```python
from build123d import *

# Parameters (mm, degrees)
F1_DEPTH  = 76.2
F1_FACE_W = 152.4
F1_FACE_H = 152.4
F2_DEPTH  = 25.4
F3_R      = 12.123607
F4_DEPTH  = 76.201
F6_DEPTH  = 28.794128
F8_DEPTH  = 25.401


with BuildPart() as f1:
    # F0 (on Front) → F1 (new body, symmetric)
    with BuildSketch(Plane.XZ):
        Polygon((-76.2, 0), (0, 0), (0, 152.4), (-25.4, 152.4), (-25.4, 28.793128), (-76.2, 28.793128), align=None)
    extrude(amount=F1_DEPTH, both=True)

    # F1_face (on face) → F2 (cut)
    with BuildSketch(Plane(origin=(0, 0, 76.2), x_dir=(0, 1, 0), z_dir=(1, 0, 0))):
        Rectangle(F1_FACE_W, F1_FACE_H)
    extrude(amount=F2_DEPTH, mode=Mode.SUBTRACT)

    # F3 (on face) → F4 (cut, through all)
    with BuildSketch(Plane.YZ):
        with Locations((0, 123.985767)):
            Circle(F3_R)
    extrude(amount=-F4_DEPTH, mode=Mode.SUBTRACT)

    # F5 (on face) → F6 (cut, through all)
    with BuildSketch(Plane.XY.offset(28.793128)):
        with BuildLine():
            Line((-63.5, 12.7), (-76.2, 12.7))
            Line((-76.2, 12.7), (-76.2, -12.7))
            Line((-76.2, -12.7), (-63.5, -12.7))
            ThreePointArc((-63.5, -12.7), (-50.8, 0), (-63.5, 12.7))
        make_face()
    extrude(amount=-F6_DEPTH, mode=Mode.SUBTRACT)

    # F7 (on face) → F8 (cut, through all)
    with BuildSketch(Plane(origin=(-25.4, 0, 0), x_dir=(0, -1, 0), z_dir=(-1, 0, 0))):
        with BuildLine():
            ThreePointArc((38.1, 152.4), (65.040768, 141.240768), (76.2, 114.3))
            Line((76.2, 114.3), (76.2, 152.4))
            Line((76.2, 152.4), (38.1, 152.4))
        make_face()
        with BuildLine():
            ThreePointArc((-76.2, 114.3), (-65.040768, 141.240768), (-38.1, 152.4))
            Line((-38.1, 152.4), (-76.2, 152.4))
            Line((-76.2, 152.4), (-76.2, 114.3))
        make_face()
    extrude(amount=-F8_DEPTH, mode=Mode.SUBTRACT)


solid = f1.part
```
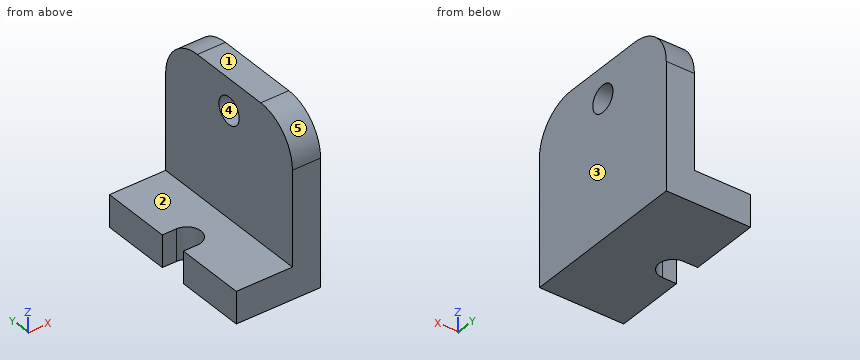
Design review of the part built by this model. Coordinates are the model's own, in mm. Face numbers are marked on the shaded views. A direction names the side the tool comes from. Coordinates: 2 decimals unless noted, no trailing zeros. Order: outer loops, then holes, each group sorted by start corner. A loop starts at its lowest first (then second) coordinate and runs counter-clockwise, first axis right, second up. Notation, with made-up numbers: M 48.25,66 L 63.25,66 A33 cw 63.25,97 Z; hole C 84,75.25 d6. An arc over 180 degrees is marked long. Answer as a JSON object with one key per item and string values. Group by question number.
1) Wall thickness on L1, parallel to Z at x = -6.75, y = 0; L2, parallel to Y at x = -62.5, z = 27.5; L3, parallel to X at y = -43.5, z = 61: over which ranges is each line inside the solid? List them lowest first.
2) Add section C-C, the plane y = -36. Write out the cut boundary in (x, z).
3) Add section A-A, the plane x = -68.5. Write out the cut boundary in (y, z), then the cut area to 3 significant figures.
4) For pin 1 (4 mm diameter, centred on y = -4.5, z = 84, fed in from -X), flat-tipped, find the tip position at first contact; note if it passes through.
5) Add section D-D, the plane x = -29.5. Write out the cut boundary in (y, z), then the cut area to 3 significant figures.
6) Mouldability with a two-part tool opening along Z and no side actions: class the marked faces 3, 4 and 5 as pulls with the +Z half, pulls with the -Z half, needs draft (parallel to the pull), parting line crosses it, or undercut.
7) Tool access review of the marked faces 1 and 2: name each direction out of +Z, -Z, +X, -X, +Y, -Y from which nothing blocks a thin tool from reaching the whole face with its end or side.
8) Add section B-B, the plane y = 0. Write out the cut boundary in (x, z), then the cut area to 3 significant figures.
Computed values:
{
 "1": {"L1": "z = 0 to 111.86, 136.11 to 152.4", "L2": "y = -76.2 to -12.66, 12.66 to 76.2", "L3": "x = -25.4 to 0"},
 "2": {"outline": "M -76.2,0 L 0,0 L 0,152.4 L -25.4,152.4 L -25.4,28.79 L -76.2,28.79 Z"},
 "3": {"outline": "M -76.2,0 L -12.7,0 L -12.7,28.79 L -76.2,28.79 Z; M 12.7,0 L 76.2,0 L 76.2,28.79 L 12.7,28.79 Z", "area": "3,660 mm^2"},
 "4": {"pin 1": "stops at x = -25.4"},
 "5": {"outline": "M -76.2,0 L 76.2,0 L 76.2,28.79 L -76.2,28.79 Z", "area": "4,390 mm^2"},
 "6": {"face 3": "needs draft", "face 4": "undercut", "face 5": "pulls with the +Z half"},
 "7": {"face 1": "+Z, +X, -X, +Y, -Y", "face 2": "+Z, -X, +Y, -Y"},
 "8": {"outline": "M -50.8,0 L 0,0 L 0,111.86 L -25.4,111.86 L -25.4,28.79 L -50.8,28.79 Z; M -25.4,136.11 L 0,136.11 L 0,152.4 L -25.4,152.4 Z", "area": "3,990 mm^2"}
}
